For this review, take the finished solid that the model builds, in its own axes (mm). Face numbers are marked on the shaded views. A direction names the side the tool comes from. Give positions to 0.01 mm unless a question says otherwise; leave off trailing zeros. Order: outer loops, then holes, each group sorted by start corner. A loop starts at its lowest first (then second) coordinate and runs counter-clockwise, first axis right, second up. Notation, with made-up numbers: (68.5, 29) -> (108.5, 29) arc R12 ccw to (108.5, 52) -> close; hole circle Ø9 at (8.5, -23). An arc over 180 degrees is marked (long way). Return JSON: item names as keys, results as strings. Group by question number.
1) To check wall thickness, follow line 1 along X through (y, z) = (14.65, 192.5); line 2 along Y through (x, z) = (19.6, 40); line 3 along Z through (x, y) = (-19.5, -10). State the ranges of each line that lie inside material, in increasing order.
2) Add section A-A (z = 192.5). Give the boundary of the cut face in (x, y), then the cut area to 3 significant figures.
3) Insertion check: P1, Ø6.5, axis at y = 10, z = 210, coming from the -X side; P2, Ø5, axis at x = 8.5, y = 10, coming from the -Z side. Each pin has a flat end and moves straight along its axis. Give the tip position at first contact, or say it passes through.
4) The part is to be moulded in two halves that separate along X. For the marked faces 1, 2 and 3, say which applies: released by +X, released by -X, zero draft, split by the parting line, or undercut.
5) Add section C-C (y = 2.75). Give the boundary of the cut face in (x, z), then the cut area to 3 significant figures.
6) Add section B-B (x = 4). Give the boundary of the cut face in (y, z).
7) Add section D-D (z = 10). Give the boundary of the cut face in (x, y), then the cut area to 3 significant figures.
8) For the marked faces 4 and 5, list the 3-axis set-ups (+Z, -Z, +X, -X, +Y, -Y) from which the entire face can be reached by the end or side of a thin tool; tool diameter is ignored.
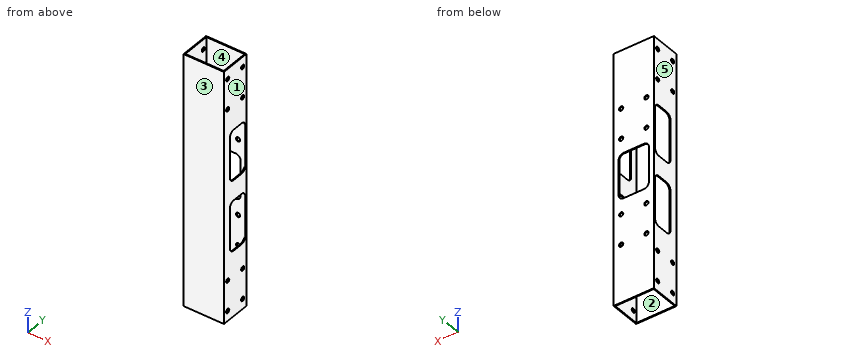
from build123d import *

# Parameters (mm, degrees)
SKETCH_1_W               = 40
SKETCH_1_H               = 30
SKETCH_1_W_2             = 38
SKETCH_1_H_2             = 28
EXTRUDE_1_DEPTH          = 250
CUT_EXTRUDE_1_DEPTH      = 252.246890528
CUT_EXTRUDE_1_DEPTH_BACK = 252.246890528
SKETCH_2_R               = 2.1
CUT_EXTRUDE_START        = 15
SKETCH_3_R               = 2.1
CUT_EXTRUDE_2_DEPTH      = 29
CUT_EXTRUDE_3_DEPTH      = 252.246890528
CUT_EXTRUDE_3_DEPTH_BACK = 252.246890528


with BuildPart() as part:
    # 草图1 → 凸台-拉伸1 (new body)
    with BuildSketch(Plane.XY):
        Rectangle(SKETCH_1_W, SKETCH_1_H)
        Rectangle(SKETCH_1_W_2, SKETCH_1_H_2, mode=Mode.SUBTRACT)
    extrude(amount=EXTRUDE_1_DEPTH)

    # 草图2 → 切除-拉伸1 (cut, two sides: drawn at the far end of the back side and taken through both)
    with BuildSketch(Plane(origin=(0, 0, 0), x_dir=(0, 0, -1), z_dir=(1, 0, 0)).offset(-CUT_EXTRUDE_1_DEPTH_BACK)):
        with Locations((-210, 10)):
            Circle(SKETCH_2_R)
        with Locations((-240, 10)):
            Circle(SKETCH_2_R)
        with Locations((-210, -10)):
            Circle(SKETCH_2_R)
        with Locations((-240, -10)):
            Circle(SKETCH_2_R)
        with Locations((-10, -10)):
            Circle(SKETCH_2_R)
        with Locations((-40, -10)):
            Circle(SKETCH_2_R)
        with Locations((-10, 10)):
            Circle(SKETCH_2_R)
        with Locations((-40, 10)):
            Circle(SKETCH_2_R)
    extrude(amount=CUT_EXTRUDE_1_DEPTH + CUT_EXTRUDE_1_DEPTH_BACK, mode=Mode.SUBTRACT)

    # 草图3 → 切除-拉伸2 (cut)
    with BuildSketch(Plane(origin=(0, 0, 0), x_dir=(1, 0, 0), z_dir=(0, 1, 0)).offset(CUT_EXTRUDE_START)):
        with Locations(Location((-12.5, -87.5, 0), (0, 0, 90))):
            Circle(SKETCH_3_R)
        with Locations(Location((12.5, -87.5, 0), (0, 0, 90))):
            Circle(SKETCH_3_R)
        with Locations(Location((-12.5, -57.5, 0), (0, 0, 90))):
            Circle(SKETCH_3_R)
        with Locations(Location((12.5, -57.5, 0), (0, 0, 90))):
            Circle(SKETCH_3_R)
        with Locations(Location((12.5, -192.5, 0), (0, 0, 90))):
            Circle(SKETCH_3_R)
        with Locations(Location((-12.5, -192.5, 0), (0, 0, 90))):
            Circle(SKETCH_3_R)
        with Locations(Location((12.5, -162.5, 0), (0, 0, 90))):
            Circle(SKETCH_3_R)
        with Locations(Location((-12.5, -162.5, 0), (0, 0, 90))):
            Circle(SKETCH_3_R)
        with BuildLine():
            Line((-10, -147.5), (10, -147.5))
            ThreePointArc((10, -147.5), (13.535533906, -146.035533906), (15, -142.5))
            Line((15, -142.5), (15, -107.5))
            ThreePointArc((15, -107.5), (13.535533906, -103.964466094), (10, -102.5))
            Line((10, -102.5), (-10, -102.5))
            ThreePointArc((-10, -102.5), (-13.535533906, -103.964466094), (-15, -107.5))
            Line((-15, -107.5), (-15, -142.5))
            ThreePointArc((-15, -142.5), (-13.535533906, -146.035533906), (-10, -147.5))
        make_face()
    extrude(amount=-CUT_EXTRUDE_2_DEPTH, mode=Mode.SUBTRACT)

    # 草图4 → 切除-拉伸3 (cut, two sides: drawn at the far end of the back side and taken through both)
    with BuildSketch(Plane(origin=(0, 0, 0), x_dir=(0, 0, -1), z_dir=(1, 0, 0)).offset(-CUT_EXTRUDE_3_DEPTH_BACK)):
        with BuildLine():
            Line((-180, -7), (-140, -7))
            ThreePointArc((-140, -7), (-136.464466094, -5.535533906), (-135, -2))
            Line((-135, -2), (-135, 8.5))
            ThreePointArc((-135, 8.5), (-136.464466094, 12.035533906), (-140, 13.5))
            Line((-140, 13.5), (-180, 13.5))
            ThreePointArc((-180, 13.5), (-183.535533906, 12.035533906), (-185, 8.5))
            Line((-185, 8.5), (-185, -2))
            ThreePointArc((-185, -2), (-183.535533906, -5.535533906), (-180, -7))
        make_face()
        with BuildLine():
            Line((-115, -2), (-115, 8.5))
            ThreePointArc((-115, 8.5), (-113.535533906, 12.035533906), (-110, 13.5))
            Line((-110, 13.5), (-70, 13.5))
            ThreePointArc((-70, 13.5), (-66.464466094, 12.035533906), (-65, 8.5))
            Line((-65, 8.5), (-65, -2))
            ThreePointArc((-65, -2), (-66.464466094, -5.535533906), (-70, -7))
            Line((-70, -7), (-110, -7))
            ThreePointArc((-110, -7), (-113.535533906, -5.535533906), (-115, -2))
        make_face()
    extrude(amount=CUT_EXTRUDE_3_DEPTH + CUT_EXTRUDE_3_DEPTH_BACK, mode=Mode.SUBTRACT)


solid = part.part
Evaluation:
{
 "1": {"line 1": "-20 to -14.6, -10.4 to 10.4, 14.6 to 20", "line 2": "-15 to -12.1, -7.9 to 7.9, 12.1 to 15", "line 3": "0 to 7.9, 12.1 to 37.9, 42.1 to 207.9, 212.1 to 237.9, 242.1 to 250"},
 "2": {"outline": "(-20, -15) -> (20, -15) -> (20, 15) -> (14.6, 15) -> (14.6, 14) -> (19, 14) -> (19, -14) -> (-19, -14) -> (-19, 14) -> (-14.6, 14) -> (-14.6, 15) -> (-20, 15) -> close; (-10.4, 14) -> (10.4, 14) -> (10.4, 15) -> (-10.4, 15) -> close", "area": "128 mm^2"},
 "3": {"P1": "x = -20", "P2": "through"},
 "4": {"face 1": "released by +X", "face 2": "undercut", "face 3": "zero draft"},
 "5": {"outline": "(-20, 0) -> (-19, 0) -> (-19, 65) -> (-20, 65) -> close; (-20, 115) -> (-19, 115) -> (-19, 135) -> (-20, 135) -> close; (-20, 185) -> (-19, 185) -> (-19, 250) -> (-20, 250) -> close; (19, 0) -> (20, 0) -> (20, 65) -> (19, 65) -> close; (19, 115) -> (20, 115) -> (20, 135) -> (19, 135) -> close; (19, 185) -> (20, 185) -> (20, 250) -> (19, 250) -> close", "area": "300 mm^2"},
 "6": {"outline": "(-15, 0) -> (-14, 0) -> (-14, 250) -> (-15, 250) -> close; (14, 0) -> (15, 0) -> (15, 102.5) -> (14, 102.5) -> close; (14, 147.5) -> (15, 147.5) -> (15, 250) -> (14, 250) -> close"},
 "7": {"outline": "(-20, -15) -> (20, -15) -> (20, -12.1) -> (19, -12.1) -> (19, -14) -> (-19, -14) -> (-19, -12.1) -> (-20, -12.1) -> close; (-20, -7.9) -> (-19, -7.9) -> (-19, 7.9) -> (-20, 7.9) -> close; (-20, 12.1) -> (-19, 12.1) -> (-19, 14) -> (19, 14) -> (19, 12.1) -> (20, 12.1) -> (20, 15) -> (-20, 15) -> close; (19, -7.9) -> (20, -7.9) -> (20, 7.9) -> (19, 7.9) -> close", "area": "119 mm^2"},
 "8": {"face 4": "+Z, -Z", "face 5": "+Z, -Z, -X, +Y, -Y"}
}
